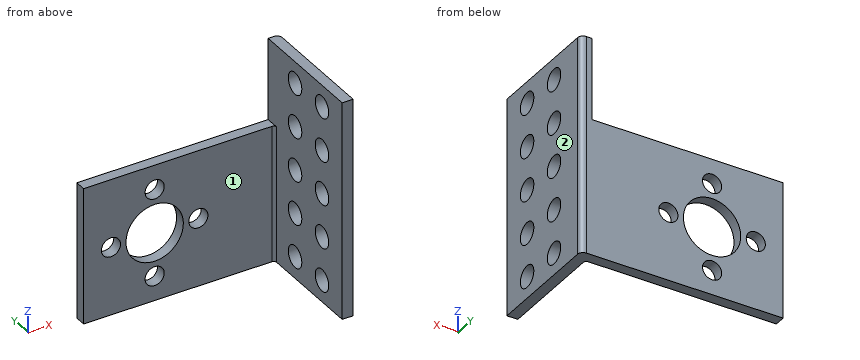
from build123d import *

# Parameters (mm, degrees)
SKETCH1_W           = 35
SKETCH1_H           = 25
SKETCH1_R           = 5.25
SKETCH1_R_2         = 1.75
BOSS_EXTRUDE1_DEPTH = 2
BOSS_EXTRUDE2_DEPTH = 2
SKETCH3_R           = 2
CUT_EXTRUDE1_DEPTH  = 59.043087444
FILLET1_R           = 1
FILLET2_R           = 0.5


with BuildPart() as part:
    # Sketch1 → Boss-Extrude1 (new body)
    with BuildSketch(Plane(origin=(0, 0, 0), x_dir=(1, 0, 0), z_dir=(0, 1, 0))):
        with Locations((17.5, -12.5)):
            Rectangle(SKETCH1_W, SKETCH1_H)
        with Locations(Location((13, -12.5, 0), (0, 0, 270))):
            Circle(SKETCH1_R, mode=Mode.SUBTRACT)
        with Locations(Location((13, -4.5, 0), (0, 0, 270))):
            Circle(SKETCH1_R_2, mode=Mode.SUBTRACT)
        with Locations(Location((21, -12.5, 0), (0, 0, 270))):
            Circle(SKETCH1_R_2, mode=Mode.SUBTRACT)
        with Locations(Location((13, -20.5, 0), (0, 0, 270))):
            Circle(SKETCH1_R_2, mode=Mode.SUBTRACT)
        with Locations(Location((5, -12.5, 0), (0, 0, 270))):
            Circle(SKETCH1_R_2, mode=Mode.SUBTRACT)
    extrude(amount=BOSS_EXTRUDE1_DEPTH)

    # Sketch2 → Boss-Extrude2 (add)
    with BuildSketch(Plane(origin=(35, 0, 0), x_dir=(0, 0, -1), z_dir=(1, 0, 0))):
        Polygon((-25, 2), (-40, 2), (-40, -20), (0, -20), (0, 2), align=None)
    extrude(amount=BOSS_EXTRUDE2_DEPTH)

    # Sketch3 → Cut-Extrude1 (cut, through all)
    with BuildSketch(Plane(origin=(37, 0, 0), x_dir=(0, 0, -1), z_dir=(1, 0, 0))):
        with Locations((-20, -6)):
            Circle(SKETCH3_R)
        with Locations((-12, -6)):
            Circle(SKETCH3_R)
        with Locations((-4, -6)):
            Circle(SKETCH3_R)
        with Locations((-28, -6)):
            Circle(SKETCH3_R)
        with Locations((-36, -6)):
            Circle(SKETCH3_R)
        with Locations((-36, -14)):
            Circle(SKETCH3_R)
        with Locations((-28, -14)):
            Circle(SKETCH3_R)
        with Locations((-20, -14)):
            Circle(SKETCH3_R)
        with Locations((-12, -14)):
            Circle(SKETCH3_R)
        with Locations((-4, -14)):
            Circle(SKETCH3_R)
    extrude(amount=-CUT_EXTRUDE1_DEPTH, mode=Mode.SUBTRACT)

    # Fillet1
    fillet1_edges = [part.edges().sort_by_distance(p)[0] for p in [
        (37, 2, 20),
    ]]
    fillet(fillet1_edges, radius=FILLET1_R)

    # Fillet2
    fillet2_edges = [part.edges().sort_by_distance(p)[0] for p in [
        (35, 0, 12.5),
    ]]
    fillet(fillet2_edges, radius=FILLET2_R)


solid = part.part
Read the model definition and answer for the solid it produces. Units are mm, in the model's axes. Face numbers are marked on the shaded views. A direction names the side the tool comes from. Round coordinates to 2 decimals unless told otherwise and drop trailing zeros. Order: outer loops, then holes, each group sorted by start corner. A loop starts at its lowest first (then second) coordinate and runs counter-clockwise, first axis right, second up.
1) Straight lines are drawn through the part: L1, parallel to Y at x = 36, z = 4; L2, parallel to X at y = 0.8, z = 12.5; L3, parallel to Y at x = 2, z = 2.5. For each, find the intervals that lie inside material, in ascending order.
2) The part is cut by section A-A on y = -6. Write down the section's boundary in (x, z), plus the area to 3 significant figures.
3) The part is cut by section B-B on z = 28. Write down the section's boundary in (x, y).
4) The part is cut by section C-C on x = 5. Write down the section's boundary in (y, z), plus the area to 3 significant figures.
5) The part is cut by section D-D on z = 13. Write down the section's boundary in (x, y), plus the area to 3 significant figures.
6) For the marked faces 1 and 2, determine the directions among +Z, -Z, +X, -X, +Y, -Y from which every point of the face is accessible in a straight line to the end or side of a thin tool.
7) Flat-ended cylindrical pins translate along their axes: pin 1 (8 mm diameter, centred on x = 14, y = -3, fed in from +Z); pin 2 (4 mm diameter, centred on x = 5, z = 12.5, fed in from -Y); pin 3 (2 mm diameter, centred on y = -1, z = 29, fed in from -X). Find the tip coordinate at first contact, or state that the pin passes through.
Resolved:
1. L1: y = -20 to -16, -12 to -8, -4 to 2
1. L2: x = 0 to 3.25, 6.75 to 7.75, 18.25 to 19.25, 22.75 to 37
1. L3: y = 0 to 2
2. outline: (35, 0) - (37, 0) - (37, 2) - (35, 2) - close; (35, 6) - (37, 6) - (37, 10) - (35, 10) - close; (35, 14) - (37, 14) - (37, 18) - (35, 18) - close; (35, 22) - (37, 22) - (37, 26) - (35, 26) - close; (35, 30) - (37, 30) - (37, 34) - (35, 34) - close; (35, 38) - (37, 38) - (37, 40) - (35, 40) - close
2. area: 40.0 mm2
3. outline: (35, -20) - (37, -20) - (37, -16) - (35, -16) - close; (35, -12) - (37, -12) - (37, -8) - (35, -8) - close; (35, -4) - (37, -4) - (37, 1) arc R1 ccw to (36, 2) - (35, 2) - close
4. outline: (0, 0) - (2, 0) - (2, 10.75) - (0, 10.75) - close; (0, 14.25) - (2, 14.25) - (2, 25) - (0, 25) - close
4. area: 43.0 mm2
5. outline: (0, 0) - (3.32, 0) - (3.32, 2) - (0, 2) - close; (6.68, 0) - (7.77, 0) - (7.77, 2) - (6.68, 2) - close; (18.23, 0) - (19.32, 0) - (19.32, 2) - (18.23, 2) - close; (22.68, 0) - (34.5, 0) arc R0.5 cw to (35, -0.5) - (35, -4.27) - (37, -4.27) - (37, 1) arc R1 ccw to (36, 2) - (22.68, 2) - close; (35, -20) - (37, -20) - (37, -15.73) - (35, -15.73) - close; (35, -12.27) - (37, -12.27) - (37, -7.73) - (35, -7.73) - close
5. area: 65.7 mm2
6. face 1: +Z, -Z, -X, -Y
6. face 2: +Z, -Z, +X, +Y, -Y
7. pin 1: stops at z = 25
7. pin 2: stops at y = 0
7. pin 3: stops at x = 35
